from build123d import *

# Parameters (mm, degrees)
F0_W     = 120
F0_H     = 100
F1_DEPTH = 10
F2_R     = 5
F3_DEPTH = 15


with BuildPart() as f1:
    # F0 (on Front) → F1 (new body)
    with BuildSketch(Plane.XZ):
        Rectangle(F0_W, F0_H)
    extrude(amount=F1_DEPTH)

    # F2 (on face) → F3 (join)
    with BuildSketch(Plane.XZ.offset(10)):
        with Locations((-41.517758, 30.551978)):
            Circle(F2_R)
        with Locations((-43.986055, -5.363304)):
            Circle(F2_R)
        with Locations((-26.031511, -41.107316)):
            Circle(F2_R)
        with Locations((17.834636, -37.677866)):
            Circle(F2_R)
        with Locations((50.760479, -2.750959)):
            Circle(F2_R)
        with Locations((20.600477, 39.609097)):
            Circle(F2_R)
    extrude(amount=F3_DEPTH)


solid = f1.part
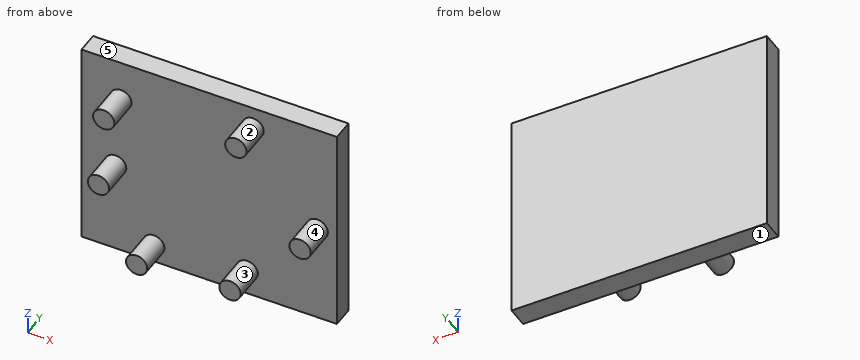
The model under review builds one solid part; all positions refer to its coordinate system, in mm. Face numbers are marked on the shaded views. A direction names the side the tool comes from. Round coordinates to 2 decimals unless told otherwise and drop trailing zeros. Order: outer loops, then holes, each group sorted by start corner. A loop starts at its lowest first (then second) coordinate and runs counter-clockwise, first axis right, second up. Notation, with made-up numbers: (60.25, 37.5) -> (66.25, 37.5) arc R14 cw to (66.25, 44.5) -> close; hole circle Ø1 at (62, 18). An arc over 180 degrees is marked (long way). Write item = value, one per line. Start each with the question number.
Item 1: Clearance check with flat-ended pins moving along their axes: pin 1 Ø2 at (x, y) = (21.5, -21.5) entering from +Z; pin 2 Ø4 at (x, z) = (30.5, 17) entering from -Y. State where each tip first meets the part, or that it passes through.
Item 2: Consider section D-D on z = 21. Write out the cut boundary in (x, y).
Item 3: Consider section B-B on z = 43. Write out the cut boundary in (x, y).
Item 4: Mouldability with a two-part tool opening along Z and no side actions: class the marked faces 3, 4 and 5 as released by +Z, released by -Z, zero draft, split by the parting line, or undercut.
Item 5: For line 1 along Y through (x, z) = (-20, 32); line 2 along Z through (x, y) = (-43, -23.5); line 3 along Z through (x, y) = (-45.5, -16.75), list the stretches that pass through material, from the lowest coordinate up.
Item 6: Consider section A-A on y = -13.25. Write out the cut boundary in (x, z), plus the area to 3 significant figures.
Item 7: Consider section C-C on x = 27.5. Write out the cut boundary in (y, z).
Item 8: For the marked faces 1 and 2, list the 3-axis set-ups (+Z, -Z, +X, -X, +Y, -Y) from which the entire face can be reached by the end or side of a thin tool; tool diameter is ignored.
Conclusion:
q1.pin_1 = 44.61
q1.pin_2 = -10
q2.outline = (-60, -10) -> (60, -10) -> (60, 0) -> (-60, 0) -> close
q3.outline = (-60, -10) -> (16.93, -10) -> (16.93, -25) -> (24.27, -25) -> (24.27, -10) -> (60, -10) -> (60, 0) -> (-60, 0) -> close
q4.face_3 = undercut
q4.face_4 = split by the parting line
q4.face_5 = released by +Z
q5.line_1 = -10 to 0
q5.line_2 = -10.27 to -0.46, 25.78 to 35.33
q5.line_3 = -10.13 to -0.6, 27.53 to 33.58
q6.outline = circle Ø10 at (-43.99, -5.36); circle Ø10 at (-41.52, 30.55); circle Ø10 at (-26.03, -41.11); circle Ø10 at (17.83, -37.68); circle Ø10 at (20.6, 39.61); circle Ø10 at (50.76, -2.75)
q6.area = 471 mm2
q7.outline = (-10, -50) -> (0, -50) -> (0, 50) -> (-10, 50) -> close
q8.face_1 = -Z, +X, -X, +Y, -Y
q8.face_2 = -Y
